Verification items for the finished model (mm, model axes). A direction names the side the tool comes from. Round coordinates to 2 decimals unless told otherwise and drop trailing zeros. Write each loop counter-clockwise with the first axis right and the second up, starting at its lowest first coordinate (ties: lowest second). Pieces come first, ordered by that corner, then holes. Notation, with made-up numbers: (-17.75, -19) - (22.25, -19) arc R16 ccw to (22.25, -6) - close; hole circle Ø6 at (-11, -4.75). An arc over 180 degrees is marked (long way). Answer as a JSON object with one key per item and string values.
```python
from build123d import *

# Parameters (mm, degrees)
CROQUIS1_R              = 1.5
SALIENTE_EXTRUIR1_DEPTH = 5


with BuildPart() as part:
    # Croquis1 → Saliente-Extruir1 (new body)
    with BuildSketch(Plane(origin=(0, 0, 0), x_dir=(1, 0, 0), z_dir=(0, 1, 0))):
        with BuildLine():
            Line((0, -3), (129.261088854, -2.336866912))
            Line((129.261088854, -2.336866912), (138.979125155, -11.494366527))
            Line((138.979125155, -11.494366527), (167.76042343, -11.494366527))
            Line((167.76042343, -11.494366527), (177.151035775, -2.091182702))
            ThreePointArc((177.151035775, -2.091182702), (176.95596642, 2.274685773), (172.610149506, 1.813453781))
            Line((172.610149506, 1.813453781), (164.264425587, -6.494366527))
            Line((164.264425587, -6.494366527), (142.859531648, -6.494366527))
            Line((142.859531648, -6.494366527), (133.197849193, 2.991093014))
            Line((133.197849193, 2.991093014), (0.470896611, 2.962812242))
            ThreePointArc((0.470896611, 2.962812242), (-2.99068861, 0.236181365), (0, -3))
        make_face()
        with Locations(Location((0, 0, 0), (0, 0, 270))):
            Circle(CROQUIS1_R, mode=Mode.SUBTRACT)
        with Locations(Location((175, 0, 0), (0, 0, 270))):
            Circle(CROQUIS1_R, mode=Mode.SUBTRACT)
    extrude(amount=SALIENTE_EXTRUIR1_DEPTH)


solid = part.part
```
Q1. Set-up check for faces 1 (the flat face through (153, 2, 11.494)), 2 (the flat face through (168.5, 2.46, 2.28)): record each of +Z, -Z, +X, -X, +Y, -Y from which the full face is reachable in a straight line by a thin tool's end or side.
Geometry check:
{"face 1": "+Z, +X, -X, +Y, -Y", "face 2": "-Z, +Y, -Y"}
Q2. Material ranges on line 1 along X through (y, z) = (3.6, 0); line 2 along X through (y, z) = (3.4, 0.5); line 3 along Z through (x, y) = (144.5, 0.6), recorded low to high. Write a range as [from, to].
Geometry check:
{"line 1": "x = [-3, -1.5], [1.5, 136.24], [170.79, 173.5], [176.5, 178]", "line 2": "x = [-2.96, -1.41], [1.41, 136.75], [170.29, 173.59], [176.41, 177.96]", "line 3": "z = [6.49, 11.49]"}
Q3. Gauge pin test, flat ends, axial feed: P1, Ø1.5, axis at y = 1.5, z = 10, coming from the -X side; P2, Ø1, axis at x = 41, y = 4.5, coming from the -Z side. Record the tip position at first contact, or that the pin passes through.
Geometry check:
{"P1": "stops at x = 136.6", "P2": "stops at z = -2.97"}
Q4. Section check B-B, the plane z = 4.5. Record the cut outline in (x, y), then the cut area to 3 significant figures.
Geometry check:
{"outline": "(131.56, 0) - (140.83, 0) - (140.83, 5) - (131.56, 5) - close; (166.27, 0) - (174.75, 0) - (174.75, 5) - (166.27, 5) - close", "area": "88.7 mm2"}
Q5. Section check A-A, the plane y = 0.8. Record the cut outline in (x, z).
Geometry check:
{"outline": "(0, 3) arc R3 ccw (long way) to (0.47, -2.96) - (133.2, -2.99) - (142.86, 6.49) - (164.26, 6.49) - (172.61, -1.81) arc R3 ccw (long way) to (177.15, 2.09) - (167.76, 11.49) - (138.98, 11.49) - (129.26, 2.34) - close; hole circle Ø3 at (0, 0); hole circle Ø3 at (175, 0)"}
Q6. Release check for a two-part mould opening along Z. For faces 3 (the flat face through (86, 5, 1)), 4 (the flat face through (138.1, 2.46, 1.82)), 5 (the cylindrical face through (0.45, 2.46, 1.43)) record: released by +Z, released by -Z, zero draft, split by the parting line, or undercut.
Geometry check:
{"face 3": "zero draft", "face 4": "released by -Z", "face 5": "undercut"}
Q7. Section check D-D, the plane x = 67. Record the cut outline in (y, z), then the cut area to 3 significant figures.
Geometry check:
{"outline": "(0, -2.98) - (5, -2.98) - (5, 2.66) - (0, 2.66) - close", "area": "28.2 mm2"}
Q8. Section check C-C, the plane x = 175. Record the cut outline in (y, z), then the cut area to 3 significant figures.
Geometry check:
{"outline": "(0, -3) - (5, -3) - (5, -1.5) - (0, -1.5) - close; (0, 1.5) - (5, 1.5) - (5, 4.25) - (0, 4.25) - close", "area": "21.2 mm2"}
